from build123d import *

# Parameters (mm, degrees)
BOSS_EXTRUDE1_DEPTH = 57.15
SKETCH4_R           = 16.51
CUT_EXTRUDE1_DEPTH  = 310.020008061
SKETCH5_W           = 49.699696275
SKETCH5_H           = 31.75
CUT_EXTRUDE2_DEPTH  = 304.425034295


with BuildPart() as part:
    # Sketch1 → Boss-Extrude1 (new body)
    with BuildSketch(Plane(origin=(0, 0, 0), x_dir=(1, 0, 0), z_dir=(0, 1, 0))):
        with BuildLine():
            Line((0, 0), (3.175, 0))
            ThreePointArc((3.175, 0), (141.2875, 80.01), (279.4, 0))
            Line((279.4, 0), (282.575, 0))
            ThreePointArc((282.575, 0), (141.2875, 94.615), (0, 0))
        make_face()
    extrude(amount=BOSS_EXTRUDE1_DEPTH)

    # Sketch4 → Cut-Extrude1 (cut, through all)
    with BuildSketch(Plane(origin=(-15.966248852, 0, -55.68092686), x_dir=(-0.9612616959383227, 0, 0.275637355816986), z_dir=(-0.275637355816986, 0, -0.9612616959383227))):
        with Locations((-122.428, 28.575)):
            Circle(SKETCH4_R)
    extrude(amount=-CUT_EXTRUDE1_DEPTH, mode=Mode.SUBTRACT)

    # Sketch5 → Cut-Extrude2 (cut, through all)
    with BuildSketch(Plane(origin=(0, 0, 0), x_dir=(1, 0, 0), z_dir=(0, 1, 0))):
        with Locations((24.849848138, 15.875)):
            Rectangle(SKETCH5_W, SKETCH5_H)
    extrude(amount=CUT_EXTRUDE2_DEPTH, mode=Mode.SUBTRACT)


solid = part.part
Can you work these out from the model? Positions are in its coordinate system, mm. A direction names the side the tool comes from. Coordinates: 2 decimals unless noted, no trailing zeros. Write each loop counter-clockwise with the first axis right and the second up, starting at its lowest first coordinate (ties: lowest second). Pieces come first, ordered by that corner, then holes. Notation, with made-up numbers: (-38, -38.5) -> (-19, -38.5) arc R18 ccw to (-19, -3.5) -> close; hole circle Ø9 at (27.25, -37). An arc over 180 degrees is marked (long way). Write item = value, one per line.
(1) For pin 1 (2 mm diameter, centred on x = 80.5, y = 20, fed in from -Z); pin 2 (10 mm diameter, centred on y = 13, z = -64.5, fed in from -X); pin 3 (10.5 mm diameter, centred on x = 23, y = 22.5, fed in from +Z), each with a flat end and sliding along its axis, tell me the tip position at first contact or that it passes through.
Verdict:
pin_1 = -82.43
pin_2 = 43.83
pin_3 = -31.75
(2) Imagine slicing it at A-A (z = -69). Please give me the cut outline in (x, y), and give its area (3 significant figures).
Verdict:
outline = (56.6, 0) -> (83.11, 0) -> (83.11, 57.15) -> (56.6, 57.15) -> close; (199.46, 0) -> (225.97, 0) -> (225.97, 57.15) -> (199.46, 57.15) -> close
area = 3,030 mm^2
(3) Imagine slicing it at C-C (x = 36). Please give me the cut outline in (y, z).
Verdict:
outline = (0, -52.55) -> (57.15, -52.55) -> (57.15, -40.22) -> (0, -40.22) -> close
(4) On a 3-axis mill with a long thin cutter (end or side, diameter ignored), from which of +Z, -Z, +X, -X, +Y, -Y can I reach the whole of each face in a straight line? I mean faces 1 (the face through (22, 28, -31.75)), 2 (the face through (150, 0, -83)). Say none if no direction works.
Verdict:
face_1 = +Z, -X, +Y, -Y
face_2 = +Z, -Z, +X, -X, -Y
(5) If I drill on probe 1 along X at (y, z) = (34.5, -46.5); probe 2 along Y at (x, z) = (105, -86); probe 3 along X at (y, z) = (49.5, -54.5), over which ranges is the centre line in solid material (lowest first)?
Verdict:
probe_1 = 29.98 to 43.58, 239 to 252.59
probe_2 = 0 to 12.21, 44.94 to 57.15
probe_3 = 38.09 to 54.85, 227.73 to 244.49
(6) Thinking about a two-plate mould opening in X: for faces 3 (the face through (115.56, 39.73, -85.31)), 4 (the face through (150, 57.15, -83)), 5 (the face through (159.12, 28.17, -79.01)), 6 (the face through (161.73, 28.17, -93.24)), which applies, +X half, -X half, draft (parallel to the pull), parting line (faces both ways), or undercut?
Verdict:
face_3 = undercut
face_4 = draft
face_5 = undercut
face_6 = parting line
